from build123d import *

# Parameters (mm, degrees)
SKETCH_1_W          = 70
SKETCH_1_H          = 30
EXTRUDE_1_DEPTH     = 5
SKETCH_2_W          = 5
SKETCH_2_H          = 30
EXTRUDE_2_DEPTH     = 75
SKETCH_3_W          = 5
SKETCH_3_H          = 30
EXTRUDE_3_DEPTH     = 65
SKETCH_4_W          = 5
SKETCH_4_H          = 30
EXTRUDE_4_DEPTH     = 40
CUT_EXTRUDE_3_REACH = 112.454
SKETCH_6_W          = 40.2
SKETCH_6_H          = 20.4
CUT_EXTRUDE_4_REACH = 112.454
SKETCH_7_W          = 40.2
SKETCH_7_H          = 20.4
CUT_EXTRUDE_5_REACH = 89.214
SKETCH_5_R          = 1.5


with BuildPart() as part:
    # 草图1 → 凸台-拉伸1 (new body)
    with BuildSketch(Plane.XY):
        with Locations((35, 15)):
            Rectangle(SKETCH_1_W, SKETCH_1_H)
    extrude(amount=EXTRUDE_1_DEPTH)

    # 草图2 → 凸台-拉伸2 (add)
    with BuildSketch(Plane.XY.offset(5)):
        with Locations((2.5, 15)):
            Rectangle(SKETCH_2_W, SKETCH_2_H)
    extrude(amount=EXTRUDE_2_DEPTH)

    # 草图3 → 凸台-拉伸3 (add)
    with BuildSketch(Plane(origin=(5, 0, 0), x_dir=(0, 0, -1), z_dir=(1, 0, 0))):
        with Locations((-77.5, 15)):
            Rectangle(SKETCH_3_W, SKETCH_3_H)
    extrude(amount=EXTRUDE_3_DEPTH)

    # 草图4 → 凸台-拉伸4 (add)
    with BuildSketch(Plane(origin=(5, 0, 0), x_dir=(0, 0, -1), z_dir=(1, 0, 0))):
        with Locations((-40, 15)):
            Rectangle(SKETCH_4_W, SKETCH_4_H)
    extrude(amount=EXTRUDE_4_DEPTH)

    # 草图6 → 切除-拉伸3 (cut, up to next)
    with BuildSketch(Plane(origin=(0, 0, 0), x_dir=(-1, 0, 0), z_dir=(0, 0, -1)), mode=Mode.PRIVATE) as cut_extrude_3_sk1:
        with Locations((-38.9, 15)):
            Rectangle(SKETCH_6_W, SKETCH_6_H)
    cut_extrude_3_tool1 = extrude(cut_extrude_3_sk1.sketch, amount=-CUT_EXTRUDE_3_REACH, mode=Mode.PRIVATE) & part.part
    add(cut_extrude_3_tool1.solids().sort_by_distance((38.9, 15, 0))[0], mode=Mode.SUBTRACT)

    # 草图7 → 切除-拉伸4 (cut, up to next)
    with BuildSketch(Plane.XY.offset(80), mode=Mode.PRIVATE) as cut_extrude_4_sk1:
        with Locations((38.9, 15)):
            Rectangle(SKETCH_7_W, SKETCH_7_H)
    cut_extrude_4_tool1 = extrude(cut_extrude_4_sk1.sketch, amount=-CUT_EXTRUDE_4_REACH, mode=Mode.PRIVATE) & part.part
    add(cut_extrude_4_tool1.solids().sort_by_distance((38.9, 15, 80))[0], mode=Mode.SUBTRACT)

    # 草图5 → 切除-拉伸5 (cut, up to next)
    with BuildSketch(Plane.XY.offset(42.5), mode=Mode.PRIVATE) as cut_extrude_5_sk1:
        with Locations((37, 15)):
            Circle(SKETCH_5_R)
    cut_extrude_5_tool1 = extrude(cut_extrude_5_sk1.sketch, amount=-CUT_EXTRUDE_5_REACH, mode=Mode.PRIVATE) & part.part
    add(cut_extrude_5_tool1.solids().sort_by_distance((37, 15, 42.5))[0], mode=Mode.SUBTRACT)


solid = part.part
Part model, mm, in its own coordinate system. A direction names the side the tool comes from. Coordinates: 2 decimals unless noted, no trailing zeros. Loops run counter-clockwise (first coordinate to the right, second up) from the corner with the lowest first, then second, coordinate; pieces in that order, holes last. Notation, with made-up numbers: M 15,11.5 L 23,11.5 A9 cw 23,15.5 Z; hole C -9.75,22.5 d6. An arc over 180 degrees is marked long. Use a Markdown table: item, result. Add a question column.
Q1. Mould opens along Y. For faces 1 (the flat face through (59, 15, 78)), 2 (the flat face through (24, 30, 40)), 3 (the flat face through (37, 29, 5)) say: +Y half, -Y half, draft (parallel to the pull), parting line (faces both ways), or undercut.
Q2. Cut at D-D (x = 54). Write the cut outline in (y, z).
Q3. Pin check, flat tips, straight feed: P1, Ø15, axis at y = 21, z = 17.5, coming from the +X side; P2, Ø2.5, axis at x = 37, y = 15, coming from the -Z side; P3, Ø1.5, axis at y = 18.5, z = 39.5, coming from the +X side. Stop position of each tip, or through.
Q4. Which spindle directions (+Z, -Z, +X, -X, +Y, -Y) get a long thin tool onto all of the face, cutting with end or side? Do faces 4 (the flat face through (45, 15, 40)), 5 (the flat face through (39, 25.2, 78)), 6 (the flat face through (18.8, 15, 2)). Say none if no direction does.
Q5. Cut at A-A (y = 15). Write the cut outline in (x, z).
Q6. Cut at C-C (x = 23). Write the cut outline in (y, z).
Q7. Cut at B-B (x = 37). Write the cut outline in (y, z), and give its area (3 significant figures).
Q8. Probe L1, parallel to Z at x = 18, y = 9.75; L2, parallel to Z at x = 61, y = 27; L3, parallel to Y at x = 37, z = 40.8. List the from-to ranges inside material, lowest first.
Worked out:
| question | item | result |
|---|---|---|
| 1 | face 1 | undercut |
| 1 | face 2 | +Y half |
| 1 | face 3 | draft |
| 2 | outline | M 0,0 L 4.8,0 L 4.8,5 L 0,5 Z; M 0,75 L 4.8,75 L 4.8,80 L 0,80 Z; M 25.2,0 L 30,0 L 30,5 L 25.2,5 Z; M 25.2,75 L 30,75 L 30,80 L 25.2,80 Z |
| 3 | P1 | stops at x = 5 |
| 3 | P2 | passes through |
| 3 | P3 | stops at x = 45 |
| 4 | face 4 | +X, +Y, -Y |
| 4 | face 5 | +Z |
| 4 | face 6 | -Z |
| 5 | outline | M 0,0 L 18.8,0 L 18.8,5 L 5,5 L 5,37.5 L 35.5,37.5 L 35.5,42.5 L 5,42.5 L 5,75 L 18.8,75 L 18.8,80 L 0,80 Z; M 38.5,37.5 L 45,37.5 L 45,42.5 L 38.5,42.5 Z; M 59,0 L 70,0 L 70,5 L 59,5 Z; M 59,75 L 70,75 L 70,80 L 59,80 Z |
| 6 | outline | M 0,0 L 4.8,0 L 4.8,5 L 0,5 Z; M 0,37.5 L 30,37.5 L 30,42.5 L 0,42.5 Z; M 0,75 L 4.8,75 L 4.8,80 L 0,80 Z; M 25.2,0 L 30,0 L 30,5 L 25.2,5 Z; M 25.2,75 L 30,75 L 30,80 L 25.2,80 Z |
| 7 | outline | M 0,0 L 4.8,0 L 4.8,5 L 0,5 Z; M 0,37.5 L 13.5,37.5 L 13.5,42.5 L 0,42.5 Z; M 0,75 L 4.8,75 L 4.8,80 L 0,80 Z; M 16.5,37.5 L 30,37.5 L 30,42.5 L 16.5,42.5 Z; M 25.2,0 L 30,0 L 30,5 L 25.2,5 Z; M 25.2,75 L 30,75 L 30,80 L 25.2,80 Z |
| 7 | area | 231 mm2 |
| 8 | L1 | z = 0 to 5, 37.5 to 42.5, 75 to 80 |
| 8 | L2 | z = 0 to 5, 75 to 80 |
| 8 | L3 | y = 0 to 13.5, 16.5 to 30 |
